Model file for the job. Use its own axes, mm. Face numbers are marked on the shaded views. A direction names the side the tool comes from. Give positions to 0.01 mm unless a question says otherwise; leave off trailing zeros. Write each loop counter-clockwise with the first axis right and the second up, starting at its lowest first coordinate (ties: lowest second). Pieces come first, ordered by that corner, then holes.
Autodesk Inventor part; units mm, degrees
ref_plane "YZ Plane" through (0, 0, 0) normal (1, 0, 0) x (0, 1, 0)
ref_plane "XZ Plane" through (0, 0, 0) normal (0, 1, 0) x (-1, 0, 0)
ref_plane "XY Plane" through (0, 0, 0) normal (0, 0, 1) x (1, 0, 0)
sketch "Sketch1" plane through (0, 0, 0) normal (0, 0, 1) x (1, 0, 0)
  line L0 (-10, 10) -> (10, 10)
  line L1 (10, 10) -> (10, -10)
  line L2 (10, -10) -> (-10, -10)
  line L3 (-10, -10) -> (-10, 10)
  line L4 (-10, 10) -> (10, -10) construction
  line L5 (10, 10) -> (-10, -10) construction
  point P0 (0, 0)
  dimension "d0" = 20
  dimension "d1" = 20
extrude "Extrusion1" add sketch "Sketch1" along normal mid plane 20
sketch "Sketch2" plane through (0, 0, 10) normal (0, 0, 1) x (1, 0, 0)
  line L0 (10, 10) -> (-10, 10)
  line L1 (-2.5, 10) -> (2.5, 10)
  line L2 (2.5, 10) -> (2.5, 5)
  line L3 (2.5, 5) -> (-2.5, 5)
  line L4 (-2.5, 5) -> (-2.5, 10)
  line L5 (-10, 10) -> (-10, -10)
  line L6 (10, -10) -> (10, 10)
  line L7 (10, 2.5) -> (5, 2.5)
  line L8 (5, 2.5) -> (5, -2.5)
  line L9 (5, -2.5) -> (10, -2.5)
  line L10 (10, -2.5) -> (10, 2.5)
  point P0 (0, 0)
  dimension "d4" = 5
  dimension "d5" = 5
  dimension "d6" = 7.5
  dimension "d7" = 5
  dimension "d8" = 5
  dimension "d9" = 7.5
extrude "Extrusion2" cut sketch "Sketch2" against normal blind 5
sketch "Sketch3" plane through (10, -10, -10) normal (1, 0, 0) x (0, 0, -1)
  line L0 (0, 20) -> (-20, 20)
  line L1 (-12.7592, 20) -> (-7.7592, 20)
  line L2 (-7.7592, 20) -> (-7.7592, 15)
  line L3 (-7.7592, 15) -> (-12.7592, 15)
  line L4 (-12.7592, 15) -> (-12.7592, 20)
  point P0 (-10, 10)
  dimension "d12" = 5
  dimension "d13" = 5
extrude "Extrusion3" cut sketch "Sketch3" against normal blind 5
sketch "Sketch8" plane through (-10, -10, 10) normal (-1, 0, 0) x (0, 0, 1)
  circle A0 centre (-10, 10) radius 2.3529
sketch "Sketch9" plane through (-10, -10, 10) normal (0, -1, 0) x (1, 0, 0)
  circle A0 centre (10, -10) radius 2.6586
sketch "Sketch10" plane through (0, 0, -10) normal (0, 0, -1) x (-1, 0, 0)
  circle A0 centre (0, 0) radius 2.2697
hole "Hole3" at (0, -10, 0) direction (0, 1, 0) diameter 4 depth 29.3 tip angle 118 counterbore diameter 8 counterbore depth 17.5
hole "Hole4" at (0, 0, -10) direction (0, 0, 1) diameter 4 depth 29.3 tip angle 118 counterbore diameter 8 counterbore depth 17.5
hole "Hole5" at (-10, 0, 0) direction (1, 0, 0) diameter 4 depth 29.3 tip angle 118 counterbore diameter 8 counterbore depth 17.5
fillet "Fillet2" radius 3 3 edges at (0, -10, -10) (-10, -10, 0) (-10, 0, -10)
properties part number "HansKube.stl"
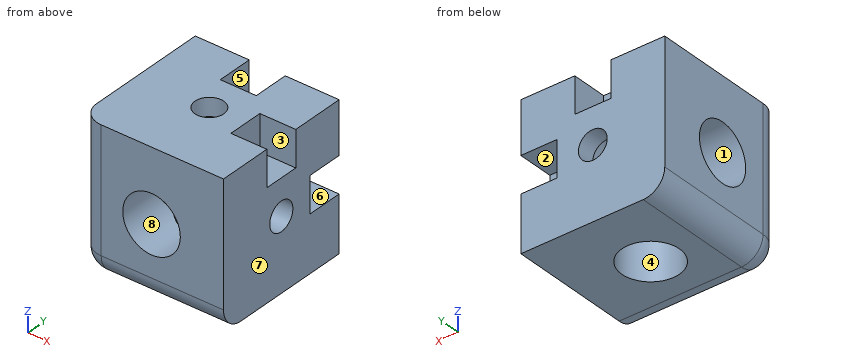
1. Slice it at A-A, the plane z = 0. Write the cut outline in (x, y), and give its area (3 significant figures).
Calculated:
outline: (-10, -7) arc R3 ccw to (-7, -10) - (-4, -10) - (-4, -4) - (-10, -4) - close; (-10, 4) - (-4, 4) - (-4, 7.5) - (-2, 7.5) - (-2, 10) - (-10, 10) - close; (2, 7.5) - (4, 7.5) - (4, 4) - (7.5, 4) - (7.5, 2) - (10, 2) - (10, 5) - (5, 5) - (5, 10) - (2, 10) - close; (4, -10) - (10, -10) - (10, -2) - (7.5, -2) - (7.5, -4) - (4, -4) - close
area: 137 mm2
2. Which spindle directions (+Z, -Z, +X, -X, +Y, -Y) get a long thin tool onto all of the face, cutting with end or side? Do the marked faces 1, 2, 3, 4 and 5. Say none if no direction does.
Calculated:
face 1: -X
face 2: +X, +Y
face 3: +Z, +X
face 4: -Z
face 5: +Z, +Y
3. Slice it at C-C, the plane y = -4.75. Write the cut outline in (x, z).
Calculated:
outline: (-10, -7) arc R3 ccw to (-7, -10) - (10, -10) - (10, 10) - (-10, 10) - close; hole circle Ø8 at (0, 0)
4. Probe probe 1 along Y at (x, z) = (0, 9.1); probe 2 along Y at (x, z) = (0, -5.25); probe 3 along Z at (x, y) = (6, 0). List the from-to ranges inside material, lowest first.
Calculated:
probe 1: y = -10 to -2, 2 to 5
probe 2: y = -10 to -4, 4 to 10
probe 3: z = -10 to -4, 4 to 5
5. Slice it at D-D, the plane z = 5.5. Write the cut outline in (x, y), and give its area (3 significant figures).
Calculated:
outline: (-10, -7) arc R3 ccw to (-7, -10) - (10, -10) - (10, -2.5) - (5, -2.5) - (5, 2.5) - (10, 2.5) - (10, 10) - (2.5, 10) - (2.5, 5) - (-2.5, 5) - (-2.5, 10) - (-10, 10) - close; hole circle Ø8 at (0, 0)
area: 298 mm2
6. Pull direction X, two halves, no side cores. Call the marked faces 6, 7 and 8: +X half, -X half, draft (parallel to the pull), parting line (faces both ways), or undercut.
Calculated:
face 6: draft
face 7: +X half
face 8: undercut
7. Pin check, flat tips, straight feed: P1, Ø4.5, axis at x = 0, y = 0, coming from the -Z side; P2, Ø2.5, axis at x = -0.5, y = 6.5, coming from the +Z side; P3, Ø6.5, axis at y = 0, z = 0, coming from the -X side. Stop position of each tip, or through.
Calculated:
P1: stops at z = 7.5
P2: stops at z = 5
P3: stops at x = 7.5
